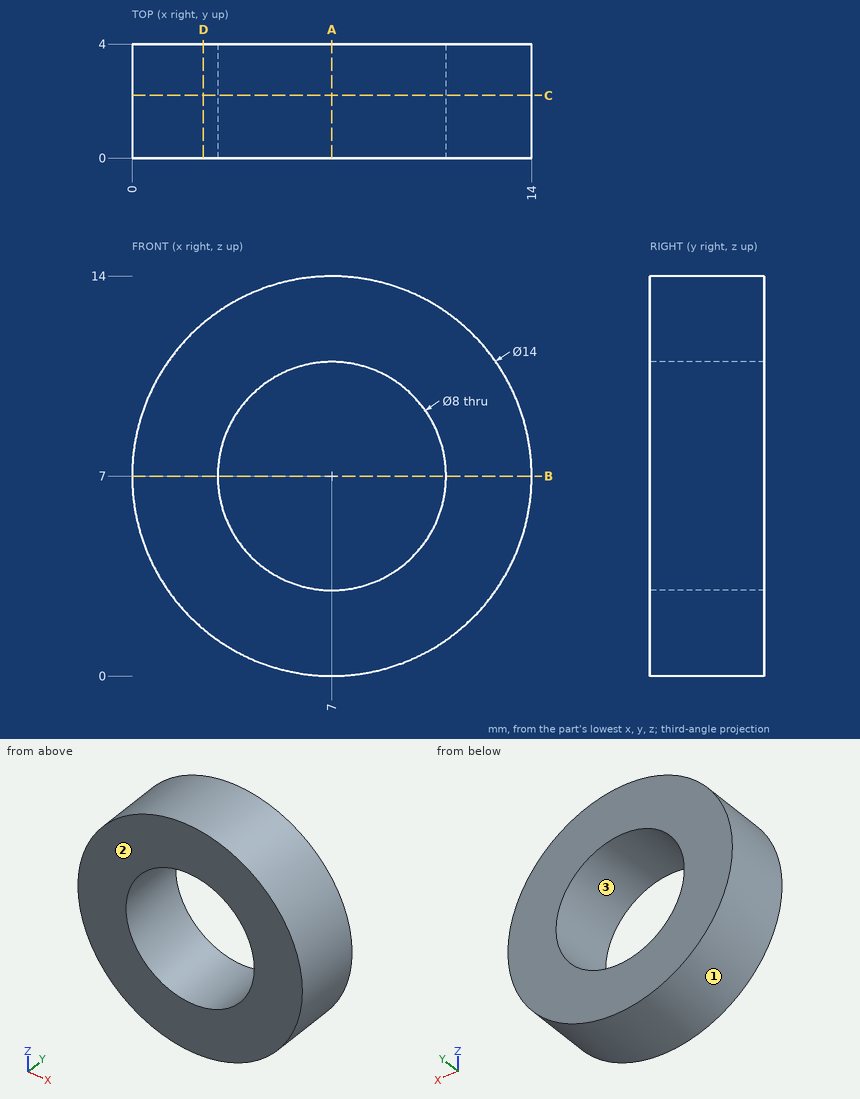
Check sheet for the drawn part. Datum: minimum x, y, z corner. Units: mm. Give positions to 0.01 mm unless a question says otherwise; leave off trailing zeros. Write each loop counter-clockwise with the first axis right and the second up, starting at its lowest first coordinate (ties: lowest second). Pieces come first, ordered by that corner, then holes.
(1) Mould release check, pull along Z, two halves, no side actions. Record for the marked faces 1, 2 and 3: +Z half, -Z half, draft (parallel to the pull), parting line (faces both ways), or undercut.
(2) Cross-section at A-A (x = 7). Enter the section's corners in (y, z).
(3) Cross-section at C-C (y = 2.2). Enter the section's corners in (x, z), plus the area to 3 significant figures.
(4) Cross-section at B-B (z = 7). Enter the section's corners in (x, y), plus the area to 3 significant figures.
(5) Gauge pin test, flat ends, axial feed: pin 1 (5 mm diameter, centred on x = 7, z = 7, fed in from +Y); pin 2 (2 mm diameter, centred on x = 10, z = 8.5, fed in from -Y); pin 3 (1 mm diameter, centred on y = 3, z = 2.5, fed in from -X). Record the tip position at first contact, or that the pin passes through.
(6) Cross-section at D-D (x = 2.5). Enter the section's corners in (y, z).
(7) Material ranges on line 1 (Z direction, x = 7, y = 2.95); line 2 (X direction, y = 2.7, z = 3.5); line 3 (X direction, y = 3.4, z = 5), recorded low to high.
Worked out:
1. face 1: parting line
1. face 2: draft
1. face 3: undercut
2. outline: (0, 0) - (4, 0) - (4, 3) - (0, 3) - close; (0, 11) - (4, 11) - (4, 14) - (0, 14) - close
3. outline: circle Ø14 at (7, 7); hole circle Ø8 at (7, 7)
3. area: 104 mm2
4. outline: (0, 0) - (3, 0) - (3, 4) - (0, 4) - close; (11, 0) - (14, 0) - (14, 4) - (11, 4) - close
4. area: 24.0 mm2
5. pin 1: passes through
5. pin 2: stops at y = 0
5. pin 3: stops at x = 1.26
6. outline: (0, 1.64) - (4, 1.64) - (4, 12.36) - (0, 12.36) - close
7. line 1: z = 0 to 3, 11 to 14
7. line 2: x = 0.94 to 5.06, 8.94 to 13.06
7. line 3: x = 0.29 to 3.54, 10.46 to 13.71
